```python
from build123d import *

# Parameters (mm, degrees)
SKETCH1_W           = 44
SKETCH1_H           = 44
BOSS_EXTRUDE1_DEPTH = 4
BOSS_EXTRUDE2_DEPTH = 12.7
SKETCH3_R           = 2.6
CUT_EXTRUDE1_DEPTH  = 63.929246102
SKETCH4_R           = 4.25
CUT_EXTRUDE2_DEPTH  = 66.177373489
FILLET1_R           = 3
FILLET2_R           = 5


with BuildPart() as part:
    # Sketch1 → Boss-Extrude1 (new body)
    with BuildSketch(Plane.XY):
        Rectangle(SKETCH1_W, SKETCH1_H)
        with BuildLine():
            Line((7, 12), (-7, 12))
            ThreePointArc((-7, 12), (-10.535533906, 10.535533906), (-12, 7))
            Line((-12, 7), (-12, -7))
            ThreePointArc((-12, -7), (-10.535533906, -10.535533906), (-7, -12))
            Line((-7, -12), (7, -12))
            ThreePointArc((7, -12), (10.535533906, -10.535533906), (12, -7))
            Line((12, -7), (12, 7))
            ThreePointArc((12, 7), (10.535533906, 10.535533906), (7, 12))
        make_face(mode=Mode.SUBTRACT)
        with BuildLine():
            Line((-19, 17.2), (-12, 17.2))
            ThreePointArc((-12, 17.2), (-10.25, 15.45), (-12, 13.7))
            Line((-12, 13.7), (-19, 13.7))
            ThreePointArc((-19, 13.7), (-20.75, 15.45), (-19, 17.2))
        make_face(mode=Mode.SUBTRACT)
        with BuildLine():
            Line((-19, -17.2), (-12, -17.2))
            ThreePointArc((-12, -17.2), (-10.25, -15.45), (-12, -13.7))
            Line((-12, -13.7), (-19, -13.7))
            ThreePointArc((-19, -13.7), (-20.75, -15.45), (-19, -17.2))
        make_face(mode=Mode.SUBTRACT)
        with BuildLine():
            Line((12, 17.2), (19, 17.2))
            ThreePointArc((19, 17.2), (20.75, 15.45), (19, 13.7))
            Line((19, 13.7), (12, 13.7))
            ThreePointArc((12, 13.7), (10.25, 15.45), (12, 17.2))
        make_face(mode=Mode.SUBTRACT)
        with BuildLine():
            Line((12, -13.7), (19, -13.7))
            ThreePointArc((19, -13.7), (20.75, -15.45), (19, -17.2))
            Line((19, -17.2), (12, -17.2))
            ThreePointArc((12, -17.2), (10.25, -15.45), (12, -13.7))
        make_face(mode=Mode.SUBTRACT)
    extrude(amount=BOSS_EXTRUDE1_DEPTH)

    # Sketch2 → Boss-Extrude2 (add)
    with BuildSketch(Plane(origin=(22, 0, 0), x_dir=(0, 0, -1), z_dir=(1, 0, 0))):
        with BuildLine():
            Line((0, 12), (-40, 12))
            Line((-40, 12), (-40, 16))
            add(Edge.make_bspline(
                [(-40, 16), (-18.32972451, 16.119369884), (-4, 22)],
                knots=[0, 0, 0, 1, 1, 1], degree=2))
            Line((-4, 22), (0, 22))
            Line((0, 22), (0, 12))
        make_face()
    boss_extrude2 = extrude(amount=BOSS_EXTRUDE2_DEPTH)

    # Sketch3 → Cut-Extrude1 (cut, through all)
    with BuildSketch(Plane.XZ.offset(-12)):
        with Locations((28.6, 35)):
            Circle(SKETCH3_R)
        with Locations((28.6, 9)):
            Circle(SKETCH3_R)
    cut_extrude1 = extrude(amount=-CUT_EXTRUDE1_DEPTH, mode=Mode.SUBTRACT)

    # Sketch4 → Cut-Extrude2 (cut, through all)
    with BuildSketch(Plane(origin=(0, 16, 0), x_dir=(-1, 0, 0), z_dir=(0, -1, 0))):
        with Locations(Location((-28.6, -9, 0), (0, 0, 180))):
            Circle(SKETCH4_R)
        with Locations(Location((-28.6, -35, 0), (0, 0, 180))):
            Circle(SKETCH4_R)
    cut_extrude2 = extrude(amount=-CUT_EXTRUDE2_DEPTH, mode=Mode.SUBTRACT)

    # Mirror1: Boss-Extrude2, Cut-Extrude1, Cut-Extrude2 across plane
    add(boss_extrude2.mirror(Plane(origin=(0, 0, 0), x_dir=(0, 0, 1), z_dir=(1, 0, 0))))
    add(cut_extrude1.mirror(Plane(origin=(0, 0, 0), x_dir=(0, 0, 1), z_dir=(1, 0, 0))), mode=Mode.SUBTRACT)
    add(cut_extrude2.mirror(Plane(origin=(0, 0, 0), x_dir=(0, 0, 1), z_dir=(1, 0, 0))), mode=Mode.SUBTRACT)

    # Fillet1
    fillet1_edges = [part.edges().sort_by_distance(p)[0] for p in [
        (34.7, 17, 0),
        (34.7, 14, 40),
        (-22, 14, 40),
        (-34.7, 17, 0),
        (-34.7, 14, 40),
        (22, 14, 40),
    ]]
    fillet(fillet1_edges, radius=FILLET1_R)

    # Fillet2
    fillet2_edges = [part.edges().sort_by_distance(p)[0] for p in [
        (22, -22, 2),
        (-22, -22, 2),
    ]]
    fillet(fillet2_edges, radius=FILLET2_R)


solid = part.part
```
Geometry: final body of the model. Coordinates: model frame, mm. A direction names the side the tool comes from. Round coordinates to 2 decimals unless told otherwise and drop trailing zeros. Write each loop counter-clockwise with the first axis right and the second up, starting at its lowest first coordinate (ties: lowest second). Pieces come first, ordered by that corner, then holes.
Item 1: Section query A-A (x = -5.5). Return loops of the section in (y, z), plus the area to 3 significant figures.
Item 2: Set-up query: faces 1 (the face through (-28, 12, 20)), 2 (the face through (22, -3, 2)), 3 (the face through (0, -12, 2)). Return all of +Z, -Z, +X, -X, +Y, -Y with unobstructed straight access to the full face (end or side cutting, diameter ignored); none if empty.
Item 3: Section query C-C (y = -15.45). Return loops of the section in (x, z), plus the area to 3 significant figures.
Item 4: Mould query, pull axis Y, two halves, no side actions, for faces 4 (the face through (0, -22, 2)), 5 (the face through (10, -11, 2)), 6 (the face through (-22, -3, 2)). Classes: +Y half, -Y half, draft (parallel to the pull), parting line (faces both ways), or undercut.
Item 5: Pin query (flat end, axial travel): P1, Ø13.5, axis at x = -28.6, z = 35, coming from the -Y side; P2, Ø3, axis at y = -6.5, z = 1.5, coming from the +X side; P3, Ø3, axis at y = -2, z = 2, coming from the -X side. Return the tip coordinate at first contact, or that it passes through.
Item 6: Section query D-D (x = 29). Give the number of separate pieces and of enclosed holes in the cut face, plus the area to 3 significant figures.
Item 7: Material intervals for L1, parallel to Z at x = 28.6, y = 13.3; L2, parallel to Z at x = -28, y = 13; L3, parallel to Y at x = 1, z = 2, sorted ascending.
Completed:
1. outline: (-22, 0) - (-12, 0) - (-12, 4) - (-22, 4) - close; (12, 0) - (22, 0) - (22, 4) - (12, 4) - close
1. area: 80.0 mm2
2. face 1: +Z, -Z, -X, -Y
2. face 2: +Z, -Z, +X, -Y
2. face 3: +Z, -Z
3. outline: (-22, 0) - (-20.75, 0) - (-20.75, 4) - (-22, 4) - close; (-10.25, 0) - (10.25, 0) - (10.25, 4) - (-10.25, 4) - close; (20.75, 0) - (22, 0) - (22, 4) - (20.75, 4) - close
3. area: 92.0 mm2
4. face 4: -Y half
4. face 5: undercut
4. face 6: draft
5. P1: stops at y = 12
5. P2: stops at x = 22
5. P3: stops at x = -22
6. separate pieces: 3
6. enclosed holes: 0
6. area: 172 mm2
7. L1: z = 0 to 6.4, 11.6 to 32.4, 37.6 to 40
7. L2: z = 0 to 6.47, 11.53 to 32.47, 37.53 to 40
7. L3: y = -22 to -12, 12 to 22
